from build123d import *

# Parameters (mm, degrees)
F0_W     = 150
F0_H     = 93
F1_DEPTH = 3
F2_W     = 20
F2_H     = 2.5
F3_DEPTH = 5
F4_R     = 4.99999
F5_R     = 1.5


# Not quite as in the source:
# - a fillet or chamfer is up to 0.001 mm smaller than in the source, because OpenCascade refuses the exact size


with BuildPart() as f1:
    # F0 (on Front) → F1 (new body)
    with BuildSketch(Plane.XZ):
        with Locations((75, 46.5)):
            Rectangle(F0_W, F0_H)
    extrude(amount=F1_DEPTH)

    # F2 (on face) → F3 (join)
    with BuildSketch(Plane.XZ.offset(3)):
        with Locations((10, 91.75)):
            Rectangle(F2_W, F2_H)
        with Locations((140, 91.75)):
            Rectangle(F2_W, F2_H)
    extrude(amount=F3_DEPTH)

    # F4 (radius 5 in the source; OpenCascade refuses exactly that, so slightly less here)
    f4_edges = [f1.edges().sort_by_distance(p)[0] for p in [
        (20, -8, 91.75),
        (130, -8, 91.75),
    ]]
    fillet(f4_edges, radius=F4_R)

    # F5
    f5_edges = [f1.edges().sort_by_distance(p)[0] for p in [
        (7.500005, -8, 93),
        (142.499995, -8, 93),
    ]]
    fillet(f5_edges, radius=F5_R)


solid = f1.part
Can you work these out from the model? Positions are in its coordinate system, mm. A direction names the side the tool comes from. Coordinates: 2 decimals unless noted, no trailing zeros. Loops run counter-clockwise (first coordinate to the right, second up) from the corner with the lowest first, then second, coordinate; pieces in that order, holes last. Notation, with made-up numbers: M -28,-2 L 24,-2 A20 ccw 24,30 Z; hole C -12,-27 d6. An arc over 180 degrees is marked long. Return JSON: item names as keys, results as strings. Group by question number.
Item 1: Thinking about a two-plate mould opening in X: for faces 1 (the cylindrical face through (132, -7, 91)), 2 (the flat face through (140, -5, 90.5)), 3 (the cylindrical face through (19, -6, 91)), 4 (the flat face through (0, -2, 50)), which applies, released by +X, released by -X, zero draft, split by the parting line, or undercut?
Item 2: Imagine slicing it at A-A (z = 63). Please give me the cut outline in (x, y), and give its area (3 significant figures).
Item 3: I'm going to push flat-ended pins straight in: pin 1 Ø1 at (x, y) = (16.5, -6.5) entering from -Z; pin 2 Ø3 at (x, z) = (71, 37) entering from -Y. Where does each tip first touch, or does it pass through?
Item 4: On a 3-axis mill with a long thin cutter (end or side, diameter ignored), from which of +Z, -Z, +X, -X, +Y, -Y can I reach the whole of each face in a straight line? I mean faces 5 (the flat face through (10, -5, 90.5)), 6 (the flat face through (74, -2, 93)). Say none if no direction works.
Item 5: Imagine slicing it at B-B (x = 72.5). Please give me the cut outline in (y, z), and give its area (3 significant figures).
Item 6: If I drill on L1, parallel to Y at x = 123, z = 75, over which ranges is the centre line in solid material (lowest first)? Write a range as from..to.
Verdict:
{
 "1": {"face 1": "undercut", "face 2": "zero draft", "face 3": "undercut", "face 4": "released by -X"},
 "2": {"outline": "M 0,-3 L 150,-3 L 150,0 L 0,0 Z", "area": "450 mm^2"},
 "3": {"pin 1": "stops at z = 90.5", "pin 2": "stops at y = -3"},
 "4": {"face 5": "-Z, +X, -X, -Y", "face 6": "+Z, +X, -X, +Y, -Y"},
 "5": {"outline": "M -3,0 L 0,0 L 0,93 L -3,93 Z", "area": "279 mm^2"},
 "6": {"L1": "y = -3..0"}
}
